from build123d import *

# Parameters (mm, degrees)
SKETCH2_R           = 2
BOSS_EXTRUDE1_DEPTH = 20.32
SKETCH3_R           = 2
CUT_EXTRUDE1_DEPTH  = 6.35
SKETCH6_R           = 4.7625
BOSS_EXTRUDE2_DEPTH = 6.35
SKETCH7_R           = 2.8
CUT_EXTRUDE3_DEPTH  = 5
CHAMFER3_SIZE       = 7.62
CHAMFER3_SIZE2      = 4.399409051
FILLET1_R           = 8


with BuildPart() as part:
    # Sketch2 → Boss-Extrude1 (new body)
    with BuildSketch(Plane.XY):
        with BuildLine():
            ThreePointArc((0, 5.08), (-5.08, 0), (0, -5.08))
            Line((0, -5.08), (18.415, -5.08))
            Line((18.415, -5.08), (18.415, 5.08))
            Line((18.415, 5.08), (0, 5.08))
        make_face()
        Circle(SKETCH2_R, mode=Mode.SUBTRACT)
    extrude(amount=BOSS_EXTRUDE1_DEPTH)

    # Sketch3 → Cut-Extrude1 (cut, symmetric)
    with BuildSketch(Plane.XY.offset(10.16)):
        with BuildLine():
            ThreePointArc((0, 5.08), (-5.08, 0), (0, -5.08))
            ThreePointArc((0, -5.08), (2.090104165, -4.630104165), (3.81, -3.360104165))
            Line((3.81, -3.360104165), (3.81, 3.360104165))
            ThreePointArc((3.81, 3.360104165), (2.090104165, 4.630104165), (0, 5.08))
        make_face()
        Circle(SKETCH3_R, mode=Mode.SUBTRACT)
        with BuildLine():
            Line((3.81, 5.08), (0, 5.08))
            ThreePointArc((0, 5.08), (2.090104165, 4.630104165), (3.81, 3.360104165))
            Line((3.81, 3.360104165), (3.81, 5.08))
        make_face()
        with BuildLine():
            Line((0, -5.08), (3.81, -5.08))
            Line((3.81, -5.08), (3.81, -3.360104165))
            ThreePointArc((3.81, -3.360104165), (2.090104165, -4.630104165), (0, -5.08))
        make_face()
    extrude(amount=CUT_EXTRUDE1_DEPTH, both=True, mode=Mode.SUBTRACT)

    # Sketch6 → Boss-Extrude2 (add)
    with BuildSketch(Plane(origin=(0, 5.08, 0), x_dir=(1, 0, 0), z_dir=(0, 1, 0))):
        with Locations((11.415, -10.16)):
            Circle(SKETCH6_R)
    extrude(amount=BOSS_EXTRUDE2_DEPTH)

    # Sketch7 → Cut-Extrude3 (cut)
    with BuildSketch(Plane(origin=(0, 11.43, 0), x_dir=(1, 0, 0), z_dir=(0, 1, 0))):
        with Locations((11.415, -10.16)):
            Circle(SKETCH7_R)
    extrude(amount=-CUT_EXTRUDE3_DEPTH, mode=Mode.SUBTRACT)

    # Chamfer3
    chamfer3_edges = [part.edges().sort_by_distance(p)[0] for p in [
        (3.81, -5.08, 10.16),
    ]]
    chamfer3_side = [part.faces().sort_by_distance(p)[0] for p in [
        (10.292029703, -5.08, 10.16),
    ]]
    chamfer(chamfer3_edges, length=CHAMFER3_SIZE, length2=CHAMFER3_SIZE2, reference=chamfer3_side[0])

    # Fillet1
    fillet1_edges = [part.edges().sort_by_distance(p)[0] for p in [
        (18.415, 0, 20.32),
        (18.415, 0, 0),
    ]]
    fillet(fillet1_edges, radius=FILLET1_R)


solid = part.part
Model file for the job. Use its own axes, mm. A direction names the side the tool comes from. Coordinates: 2 decimals unless noted, no trailing zeros. Write each loop counter-clockwise with the first axis right and the second up, starting at its lowest first coordinate (ties: lowest second). Pieces come first, ordered by that corner, then holes. Notation, with made-up numbers: (76.5, 4) - (102.5, 4) arc R7 ccw to (102.5, 8) - close; hole circle Ø2 at (-28.5, 68.25). An arc over 180 degrees is marked (long way). Write each question's results on one line, items separated by ' | '. Start each with the question number.
1) Probe line 1 along Z through (x, y) = (2, -2.5); line 2 along Y through (x, z) = (7.25, 16.75); line 3 along X through (y, z) = (4.75, 8) (3 decimals). List the from-to ranges inside material, lowest first. Write a range as from..to.
2) Cut at C-C (y = -3.5). Write the cut outline in (x, z) (3 decimals), then the cut area to 3 significant figures.
3) 3-axis set-ups, long thin cutter, end or side, ignore diameter. For faces 1 (the face through (3.81, 2, 10)), 2 (the face through (3, 0, 20.32)), 3 (the face through (12.92, 8.96, 7.8)), 4 (the face through (1, -2, 16.51)): which of +Z, -Z, +X, -X, +Y, -Y reach the whole face in a straight line?
4) Cut at B-B (z = 10.16). Write the cut outline in (x, y) (1 decimal).
5) Cut at D-D (x = 8). Write the cut outline in (y, z), then the cut area to 3 significant figures.
6) Cut at A-A (y = 0). Write the cut outline in (x, z) (3 decimals), then the cut area to 3 significant figures.
7) Mould opens along Z. For faces 5 (the face through (16.01, 0.07, 2.28)), 6 (the face through (7.57, -2.85, 10.07)), 7 (the face through (7.636, 8.211, 13.058)), 8 (the face through (-5.08, 0.11, 1.88)) say: pulls with the +Z half, pulls with the -Z half, needs draft (parallel to the pull), parting line crosses it, or undercut.
8) Flat gauge pins, fed straight in: P1, Ø6, axis at x = 13.5, y = 3, coming from the -Z side; P2, Ø3, axis at y = 3.5, z = 11, coming from the -X side; P3, Ø4, axis at y = 9.5, z = 5.5, coming from the -X side. Where does each tip first touch, or does it go through?
Returned:
1) line 1: 0..3.81, 16.51..20.32 | line 2: -5.08..5.08 | line 3: 3.81..18.415
2) outline: (-3.682, 0) - (10.415, 0) arc R8 ccw to (18.415, 8) - (18.415, 12.32) arc R8 ccw to (10.415, 20.32) - (-3.682, 20.32) - (-3.682, 16.51) - (8.693, 16.51) - (8.693, 3.81) - (-3.682, 3.81) - close | area: 264 mm^2
3) face 1: -X, +Y, -Y | face 2: +Z, +X, -X, +Y, -Y | face 3: +Y | face 4: -X, -Y
4) outline: (3.8, -0.7) - (11.4, -5.1) - (18.4, -5.1) - (18.4, 5.1) - (16.2, 5.1) - (16.2, 11.4) - (14.2, 11.4) - (14.2, 6.4) - (8.6, 6.4) - (8.6, 11.4) - (6.7, 11.4) - (6.7, 5.1) - (3.8, 5.1) - close
5) outline: (-5.08, 0) - (5.08, 0) - (5.08, 6.84) - (11.43, 6.84) - (11.43, 13.48) - (5.08, 13.48) - (5.08, 20.32) - (-5.08, 20.32) - (-5.08, 16.51) - (-3.1, 16.51) - (-3.1, 3.81) - (-5.08, 3.81) - close | area: 223 mm^2
6) outline: (-5.08, 0) - (-2, 0) - (-2, 3.81) - (-5.08, 3.81) - close; (-5.08, 16.51) - (-2, 16.51) - (-2, 20.32) - (-5.08, 20.32) - close; (2, 0) - (10.415, 0) arc R8 ccw to (18.415, 8) - (18.415, 12.32) arc R8 ccw to (10.415, 20.32) - (2, 20.32) - (2, 16.51) - (3.81, 16.51) - (3.81, 3.81) - (2, 3.81) - close | area: 307 mm^2
7) face 5: pulls with the -Z half | face 6: undercut | face 7: parting line crosses it | face 8: needs draft
8) P1: z = 0 | P2: x = 3.81 | P3: x = 7.46
